Geometry check sheet. Reference: the model listing, model coordinates, mm. A direction names the side the tool comes from. Coordinates: 2 decimals unless noted, no trailing zeros. One line per item, written item: value. Start each with the question number.
1) Thickness scan on L1, parallel to Y at x = -7.75, z = 138; L2, parallel to Y at x = 0, z = 226; L3, parallel to Y at x = 8.5, z = 193. Record the ranges inside material, lowest first. Write a range as from..to.
2) Draft check along Y on faces 4 (the flat face through (0, -6.1, 148)), 5 (the flat face through (0, 13.9, 148)), 6 (the flat face through (0, -13.9, 148)), 7 (the flat face through (-10, 0, 148)). Enter one of: pulls with the +Y half, pulls with the -Y half, needs draft (parallel to the pull), parting line crosses it, or undercut.
3) Access from +Z, -Z, +X, -X, +Y, -Y to the whole of each face (thin tool, end or side, straight path). Record for faces 1 (the flat face through (-8.2, 0, 148)), 2 (the flat face through (3.9, 10, 148)), 3 (the flat face through (-3.9, -10, 148)).
4) Sectioned sample at A-A, the plane z = 257. State how many separate pieces and enclosed holes the cut face has, then the cut area to 3 significant figures.
5) Go/stop test with flat-tipped pins: P1, Ø1.5, axis at x = -4.5, z = 81.5, coming from the +Y side; P2, Ø8, axis at x = -0.5, z = 262, coming from the -Y side; P3, Ø4.5, axis at x = -1, z = 135, coming from the +Y side; P4, Ø0.6, axis at y = -6, z = 118.5, coming from the -X side. Record where each tip stops, or that it passes through.
```python
from build123d import *

# Parameters (mm, degrees)
SKETCH1_R           = 2.1
BOSS_EXTRUDE1_DEPTH = 300


with BuildPart() as part:
    # Sketch1 → Boss-Extrude1 (new body)
    with BuildSketch(Plane.XY):
        with BuildLine():
            ThreePointArc((10, 19.5), (9.853553391, 19.853553391), (9.5, 20))
            Line((9.5, 20), (5.049211356, 20))
            Line((5.049211356, 20), (3.419922035, 18.370710678))
            ThreePointArc((3.419922035, 18.370710678), (3.398244759, 18.261731657), (3.490632713, 18.2))
            Line((3.490632713, 18.2), (5.4, 18.2))
            ThreePointArc((5.4, 18.2), (5.470710678, 18.170710678), (5.5, 18.1))
            Line((5.5, 18.1), (5.5, 16.602081528))
            ThreePointArc((5.5, 16.602081528), (5.492387953, 16.563813185), (5.470710678, 16.53137085))
            Line((5.470710678, 16.53137085), (2.839339828, 13.9))
            Line((2.839339828, 13.9), (-2.839339828, 13.9))
            Line((-2.839339828, 13.9), (-5.470710678, 16.53137085))
            ThreePointArc((-5.470710678, 16.53137085), (-5.492387953, 16.563813185), (-5.5, 16.602081528))
            Line((-5.5, 16.602081528), (-5.5, 18.1))
            ThreePointArc((-5.5, 18.1), (-5.470710678, 18.170710678), (-5.4, 18.2))
            Line((-5.4, 18.2), (-3.490632713, 18.2))
            ThreePointArc((-3.490632713, 18.2), (-3.398244759, 18.261731657), (-3.419922035, 18.370710678))
            Line((-3.419922035, 18.370710678), (-5.049211356, 20))
            Line((-5.049211356, 20), (-9.5, 20))
            ThreePointArc((-9.5, 20), (-9.853553391, 19.853553391), (-10, 19.5))
            Line((-10, 19.5), (-10, 15.049211356))
            Line((-10, 15.049211356), (-8.370710678, 13.419922035))
            ThreePointArc((-8.370710678, 13.419922035), (-8.261731657, 13.398244759), (-8.2, 13.490632713))
            Line((-8.2, 13.490632713), (-8.2, 15.4))
            ThreePointArc((-8.2, 15.4), (-8.170710678, 15.470710678), (-8.1, 15.5))
            Line((-8.1, 15.5), (-6.602081528, 15.5))
            ThreePointArc((-6.602081528, 15.5), (-6.563813185, 15.492387953), (-6.53137085, 15.470710678))
            Line((-6.53137085, 15.470710678), (-3.9, 12.839339828))
            Line((-3.9, 12.839339828), (-3.9, 7.160660172))
            Line((-3.9, 7.160660172), (-6.53137085, 4.529289322))
            ThreePointArc((-6.53137085, 4.529289322), (-6.563813185, 4.507612047), (-6.602081528, 4.5))
            Line((-6.602081528, 4.5), (-8.1, 4.5))
            ThreePointArc((-8.1, 4.5), (-8.170710678, 4.529289322), (-8.2, 4.6))
            Line((-8.2, 4.6), (-8.2, 6.509367287))
            ThreePointArc((-8.2, 6.509367287), (-8.261731657, 6.601755241), (-8.370710678, 6.580077965))
            Line((-8.370710678, 6.580077965), (-10, 4.950788644))
            Line((-10, 4.950788644), (-10, -4.950788644))
            Line((-10, -4.950788644), (-8.370710678, -6.580077965))
            ThreePointArc((-8.370710678, -6.580077965), (-8.261731657, -6.601755241), (-8.2, -6.509367287))
            Line((-8.2, -6.509367287), (-8.2, -4.6))
            ThreePointArc((-8.2, -4.6), (-8.170710678, -4.529289322), (-8.1, -4.5))
            Line((-8.1, -4.5), (-6.602081528, -4.5))
            ThreePointArc((-6.602081528, -4.5), (-6.563813185, -4.507612047), (-6.53137085, -4.529289322))
            Line((-6.53137085, -4.529289322), (-3.9, -7.160660172))
            Line((-3.9, -7.160660172), (-3.9, -10))
            Line((-3.9, -10), (-3.9, -12.839339828))
            Line((-3.9, -12.839339828), (-6.53137085, -15.470710678))
            ThreePointArc((-6.53137085, -15.470710678), (-6.563813185, -15.492387953), (-6.602081528, -15.5))
            Line((-6.602081528, -15.5), (-8.1, -15.5))
            ThreePointArc((-8.1, -15.5), (-8.170710678, -15.470710678), (-8.2, -15.4))
            Line((-8.2, -15.4), (-8.2, -13.490632713))
            ThreePointArc((-8.2, -13.490632713), (-8.261731657, -13.398244759), (-8.370710678, -13.419922035))
            Line((-8.370710678, -13.419922035), (-10, -15.049211356))
            Line((-10, -15.049211356), (-10, -19.5))
            ThreePointArc((-10, -19.5), (-9.853553391, -19.853553391), (-9.5, -20))
            Line((-9.5, -20), (-5.049211356, -20))
            Line((-5.049211356, -20), (-3.419922035, -18.370710678))
            ThreePointArc((-3.419922035, -18.370710678), (-3.398244759, -18.261731657), (-3.490632713, -18.2))
            Line((-3.490632713, -18.2), (-5.4, -18.2))
            ThreePointArc((-5.4, -18.2), (-5.470710678, -18.170710678), (-5.5, -18.1))
            Line((-5.5, -18.1), (-5.5, -16.602081528))
            ThreePointArc((-5.5, -16.602081528), (-5.492387953, -16.563813185), (-5.470710678, -16.53137085))
            Line((-5.470710678, -16.53137085), (-2.839339828, -13.9))
            Line((-2.839339828, -13.9), (2.839339828, -13.9))
            Line((2.839339828, -13.9), (5.470710678, -16.53137085))
            ThreePointArc((5.470710678, -16.53137085), (5.492387953, -16.563813185), (5.5, -16.602081528))
            Line((5.5, -16.602081528), (5.5, -18.1))
            ThreePointArc((5.5, -18.1), (5.470710678, -18.170710678), (5.4, -18.2))
            Line((5.4, -18.2), (3.490632713, -18.2))
            ThreePointArc((3.490632713, -18.2), (3.398244759, -18.261731657), (3.419922035, -18.370710678))
            Line((3.419922035, -18.370710678), (5.049211356, -20))
            Line((5.049211356, -20), (9.5, -20))
            ThreePointArc((9.5, -20), (9.853553391, -19.853553391), (10, -19.5))
            Line((10, -19.5), (10, -15.049211356))
            Line((10, -15.049211356), (8.370710678, -13.419922035))
            ThreePointArc((8.370710678, -13.419922035), (8.261731657, -13.398244759), (8.2, -13.490632713))
            Line((8.2, -13.490632713), (8.2, -15.4))
            ThreePointArc((8.2, -15.4), (8.170710678, -15.470710678), (8.1, -15.5))
            Line((8.1, -15.5), (6.602081528, -15.5))
            ThreePointArc((6.602081528, -15.5), (6.563813185, -15.492387953), (6.53137085, -15.470710678))
            Line((6.53137085, -15.470710678), (3.9, -12.839339828))
            Line((3.9, -12.839339828), (3.9, -10))
            Line((3.9, -10), (3.9, -7.160660172))
            Line((3.9, -7.160660172), (6.53137085, -4.529289322))
            ThreePointArc((6.53137085, -4.529289322), (6.563813185, -4.507612047), (6.602081528, -4.5))
            Line((6.602081528, -4.5), (8.1, -4.5))
            ThreePointArc((8.1, -4.5), (8.170710678, -4.529289322), (8.2, -4.6))
            Line((8.2, -4.6), (8.2, -6.509367287))
            ThreePointArc((8.2, -6.509367287), (8.261731657, -6.601755241), (8.370710678, -6.580077965))
            Line((8.370710678, -6.580077965), (10, -4.950788644))
            Line((10, -4.950788644), (10, 4.950788644))
            Line((10, 4.950788644), (8.370710678, 6.580077965))
            ThreePointArc((8.370710678, 6.580077965), (8.261731657, 6.601755241), (8.2, 6.509367287))
            Line((8.2, 6.509367287), (8.2, 4.6))
            ThreePointArc((8.2, 4.6), (8.170710678, 4.529289322), (8.1, 4.5))
            Line((8.1, 4.5), (6.602081528, 4.5))
            ThreePointArc((6.602081528, 4.5), (6.563813185, 4.507612047), (6.53137085, 4.529289322))
            Line((6.53137085, 4.529289322), (3.9, 7.160660172))
            Line((3.9, 7.160660172), (3.9, 12.839339828))
            Line((3.9, 12.839339828), (6.53137085, 15.470710678))
            ThreePointArc((6.53137085, 15.470710678), (6.563813185, 15.492387953), (6.602081528, 15.5))
            Line((6.602081528, 15.5), (8.1, 15.5))
            ThreePointArc((8.1, 15.5), (8.170710678, 15.470710678), (8.2, 15.4))
            Line((8.2, 15.4), (8.2, 13.490632713))
            ThreePointArc((8.2, 13.490632713), (8.261731657, 13.398244759), (8.370710678, 13.419922035))
            Line((8.370710678, 13.419922035), (10, 15.049211356))
            Line((10, 15.049211356), (10, 19.5))
        make_face()
        with Locations((0, -10)):
            Circle(SKETCH1_R, mode=Mode.SUBTRACT)
        Polygon((-5.735302207, 3.204037621), (-2.839339828, 6.1), (2.839339828, 6.1), (5.735302207, 3.204037621), (8.2, 3.204037621), (8.2, -3.117547571), (5.735302207, -3.117547571), (2.839339828, -6.1), (-2.839339828, -6.1), (-5.735302207, -3.117547571), (-8.2, -3.117547571), (-8.2, 3.204037621), align=None, mode=Mode.SUBTRACT)
        with Locations((0, 10)):
            Circle(SKETCH1_R, mode=Mode.SUBTRACT)
    extrude(amount=BOSS_EXTRUDE1_DEPTH)


solid = part.part
```
Final values:
1. L1: y = -20..-15.5, -4.5..-3.12, 3.2..4.5, 15.5..20
1. L2: y = -13.9..-12.1, -7.9..-6.1, 6.1..7.9, 12.1..13.9
1. L3: y = -20..-13.55, -6.45..6.45, 13.55..20
2. face 4: undercut
2. face 5: pulls with the +Y half
2. face 6: pulls with the -Y half
2. face 7: needs draft
3. face 1: +Z, -Z
3. face 2: +Z, -Z, +X
3. face 3: +Z, -Z, -X
4. separate pieces: 1
4. enclosed holes: 3
4. area: 287 mm^2
5. P1: stops at y = 20
5. P2: stops at y = -19.45
5. P3: stops at y = 14.31
5. P4: stops at x = -9.25
